from build123d import *

# Parameters (mm, degrees)
SKETCH1_W                  = 88.9
SKETCH1_H                  = 203.2
BOSS_EXTRUDE1_DEPTH        = 3.175
F_1_2_0_5_DIAMETER_HOLE1_D = 12.7


with BuildPart() as part:
    # Sketch1 → Boss-Extrude1 (new, symmetric)
    with BuildSketch(Plane.XY):
        Rectangle(SKETCH1_W, SKETCH1_H)
    extrude(amount=BOSS_EXTRUDE1_DEPTH, both=True)

    # 1/2 (0.5) Diameter Hole1 (through all)
    with Locations(Plane.XY.offset(3.175)):
        with Locations((0, 0)):
            Hole(F_1_2_0_5_DIAMETER_HOLE1_D / 2)


solid = part.part
Could you check a few things on this model? Use its own coordinates, in mm. Give positions to 0.01 mm unless a question says otherwise; leave off trailing zeros. Write each loop counter-clockwise with the first axis right and the second up, starting at its lowest first coordinate (ties: lowest second). Pieces come first, ordered by that corner, then holes. Notation, with made-up numbers: (7, -29) - (16, -29) arc R25 ccw to (16, -10) - close; hole circle Ø3 at (18, -28). An arc over 180 degrees is marked (long way). Use CSV: the item, a comma, the result in double quotes. Start each with the question number.
Item 1: If we mould it in two halves opening along X, with no side actions, what happens to faces 1 (the face through (1.38, -6.2, -0.04)), 2 (the face through (44.45, -1, 0)), 3 (the face through (-1, 101.6, 0))? For each: pulls with the +X half, pulls with the -X half, needs draft (parallel to the pull), parting line crosses it, or undercut.
Item 2: I want a section at A-A, the plane y = 0. Please give me the cut outline in (x, z) (3 decimals), then the cut area to 3 significant figures.
Item 3: If I drill on line 1 along Y through (x, z) = (0, 1.5); line 2 along X through (y, z) = (-5, 0.5); line 3 along Y through (x, z) = (-4.5, 1.75), over which ranges is the centre line in solid material (lowest first)?
Item 4: I want a section at B-B, the plane x = 0. Please give me the cut outline in (y, z) (3 decimals), then the cut area to 3 significant figures.
Findings:
1,face 1,"undercut"
1,face 2,"pulls with the +X half"
1,face 3,"needs draft"
2,outline,"(-44.45, -3.175) - (-6.35, -3.175) - (-6.35, 3.175) - (-44.45, 3.175) - close; (6.35, -3.175) - (44.45, -3.175) - (44.45, 3.175) - (6.35, 3.175) - close"
2,area,"484 mm2"
3,line 1,"y = -101.6 to -6.35, 6.35 to 101.6"
3,line 2,"x = -44.45 to -3.91, 3.91 to 44.45"
3,line 3,"y = -101.6 to -4.48, 4.48 to 101.6"
4,outline,"(-101.6, -3.175) - (-6.35, -3.175) - (-6.35, 3.175) - (-101.6, 3.175) - close; (6.35, -3.175) - (101.6, -3.175) - (101.6, 3.175) - (6.35, 3.175) - close"
4,area,"1,210 mm2"
